The model under review builds one solid part; all positions refer to its coordinate system, in mm. Face numbers are marked on the shaded views. A direction names the side the tool comes from. Round coordinates to 2 decimals unless told otherwise and drop trailing zeros. Order: outer loops, then holes, each group sorted by start corner. A loop starts at its lowest first (then second) coordinate and runs counter-clockwise, first axis right, second up. Notation, with made-up numbers: M -11.75,-21 L 40.25,-21 A21 cw 40.25,-12 Z; hole C -24,43.5 d1. An arc over 180 degrees is marked long. Answer as a JSON object with one key per item and string values. Group by question number.
1. Clearance check with flat-ended pins moving along their axes: P1, Ø6, axis at x = 13.5, y = 17.5, coming from the +Z side; P2, Ø2, axis at x = -0.5, z = 22, coming from the +Y side. State where each tip first meets the part, or that it passes through.
2. Machinability: for the marked faces 1 and 2, which of the approach directions +Z, -Z, +X, -X, +Y, -Y give a long, thin tool a straight path to every point of the face, cutting with its end or side? Answer none if there is none.
3. Add section A-A on x = -7. State the section outline as (y, z) points, and give its area (3 significant figures).
4. Add section C-C on x = 8.66. State the section outline as (y, z) points.
5. Add section D-D on x = 2.5. State the section outline as (y, z) points, and give its area (3 significant figures).
6. Add section B-B on y = 24. State the section outline as (x, z) points, and give its area (3 significant figures).
7. Mouldability with a two-part tool opening along X and no side actions: class the marked faces 3, 4, 5 and 6 as released by +X, released by -X, zero draft, split by the parting line, or undercut.
8. To check wall thickness, follow probe 1 along Y at (x, z) = (8.66, 24.5); probe 2 along Y at (x, z) = (-13.5, -23); probe 3 along Z at (x, y) = (5.5, 21.5). State the ranges of each line that lie inside material, in increasing order. Write a range as [from, to].
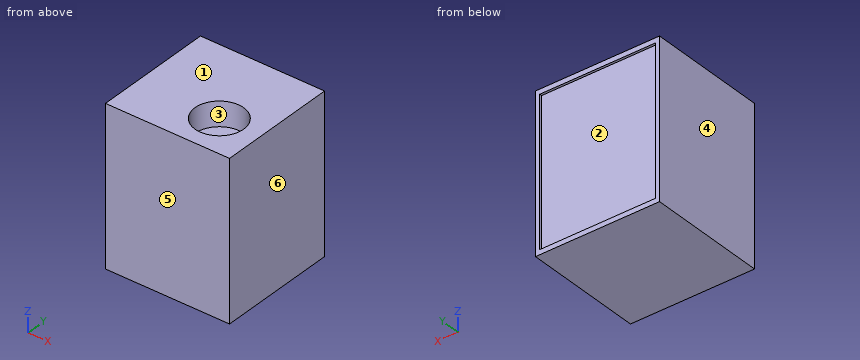
```python
from build123d import *

# Parameters (mm, degrees)
SKETCH1_W           = 51
SKETCH1_H           = 64.5
BOSS_EXTRUDE1_DEPTH = 49.4
SKETCH2_R           = 10
CUT_EXTRUDE1_DEPTH  = 10
SKETCH3_W           = 47.55649051
SKETCH3_H           = 60.50962022
CUT_EXTRUDE2_DEPTH  = 1


with BuildPart() as part:
    # Sketch1 → Boss-Extrude1 (new body)
    with BuildSketch(Plane(origin=(0, 0, 0), x_dir=(1, 0, 0), z_dir=(0, 1, 0))):
        Rectangle(SKETCH1_W, SKETCH1_H)
    extrude(amount=BOSS_EXTRUDE1_DEPTH)

    # Sketch2 → Cut-Extrude1 (cut)
    with BuildSketch(Plane.XY.offset(32.25)):
        with Locations((8.66, 16)):
            Circle(SKETCH2_R)
    extrude(amount=-CUT_EXTRUDE1_DEPTH, mode=Mode.SUBTRACT)

    # Sketch3 → Cut-Extrude2 (cut)
    with BuildSketch(Plane(origin=(0, 49.4, 0), x_dir=(1, 0, 0), z_dir=(0, 1, 0))):
        Rectangle(SKETCH3_W, SKETCH3_H)
    extrude(amount=-CUT_EXTRUDE2_DEPTH, mode=Mode.SUBTRACT)


solid = part.part
```
Recorded:
{
 "1": {"P1": "stops at z = 22.25", "P2": "stops at y = 48.4"},
 "2": {"face 1": "+Z, +X, -X, +Y, -Y", "face 2": "+Y"},
 "3": {"outline": "M 0,-32.25 L 49.4,-32.25 L 49.4,-30.25 L 48.4,-30.25 L 48.4,30.25 L 49.4,30.25 L 49.4,32.25 L 0,32.25 Z", "area": "3,130 mm²"},
 "4": {"outline": "M 0,-32.25 L 49.4,-32.25 L 49.4,-30.25 L 48.4,-30.25 L 48.4,30.25 L 49.4,30.25 L 49.4,32.25 L 26,32.25 L 26,22.25 L 6,22.25 L 6,32.25 L 0,32.25 Z"},
 "5": {"outline": "M 0,-32.25 L 49.4,-32.25 L 49.4,-30.25 L 48.4,-30.25 L 48.4,30.25 L 49.4,30.25 L 49.4,32.25 L 23.88,32.25 L 23.88,22.25 L 8.12,22.25 L 8.12,32.25 L 0,32.25 Z", "area": "2,970 mm²"},
 "6": {"outline": "M -25.5,-32.25 L 25.5,-32.25 L 25.5,32.25 L 14.66,32.25 L 14.66,22.25 L 2.66,22.25 L 2.66,32.25 L -25.5,32.25 Z", "area": "3,170 mm²"},
 "7": {"face 3": "undercut", "face 4": "released by -X", "face 5": "zero draft", "face 6": "released by +X"},
 "8": {"probe 1": "y = [0, 6], [26, 48.4]", "probe 2": "y = [0, 48.4]", "probe 3": "z = [-32.25, 22.25]"}
}
